Geometry: final body of the model. Coordinates: model frame, mm. Face numbers are marked on the shaded views. Round coordinates to 2 decimals unless told otherwise and drop trailing zeros. Write each loop counter-clockwise with the first axis right and the second up, starting at its lowest first coordinate (ties: lowest second). Pieces come first, ordered by that corner, then holes. Notation, with made-up numbers: (52.25, -34.5) - (58.25, -34.5) arc R20 cw to (58.25, -3.5) - close; hole circle Ø9 at (-27.5, 27.25). An arc over 180 degrees is marked (long way). Use a Markdown table: item, result. Add a question column.
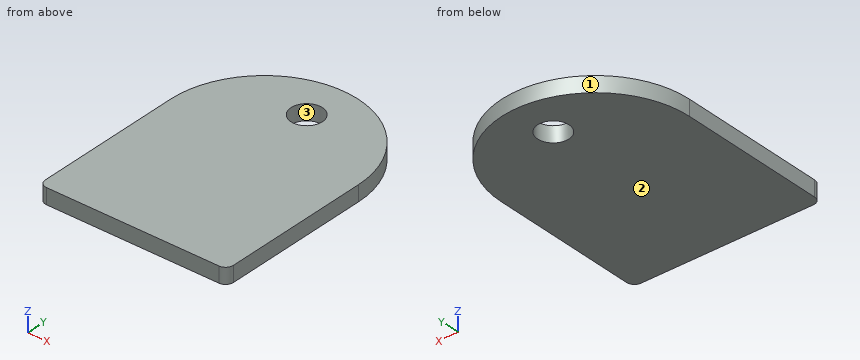
Autodesk Inventor part; units mm, degrees
ref_plane "YZ Plane" through (0, 0, 0) normal (1, 0, 0) x (0, 1, 0)
ref_plane "XZ Plane" through (0, 0, 0) normal (0, 1, 0) x (-1, 0, 0)
ref_plane "XY Plane" through (0, 0, 0) normal (0, 0, 1) x (1, 0, 0)
sketch "Sketch1" plane through (0, 0, 0) normal (0, 0, 1) x (1, 0, 0)
  circle A0 centre (-9.1291, -65.9913) radius 6.35
  line L0 (3.5709, -48.3129) -> (3.5709, -48.3129)
  line L1 (28.9709, -86.4129) -> (28.9709, -146.7379)
  line L2 (25.7959, -149.9129) -> (-44.0541, -149.9129)
  line L3 (-47.2291, -146.7379) -> (-47.2291, -86.4129)
  arc A1 (25.7959, -149.9129) -> (28.9709, -146.7379) centre (25.7959, -146.7379) ccw
  arc A2 (-47.2291, -146.7379) -> (-44.0541, -149.9129) centre (-44.0541, -146.7379) ccw
  line L4 (-9.1291, -48.3129) -> (-9.1291, -48.3129)
  arc A3 (-9.1291, -48.3129) -> (-47.2291, -86.4129) centre (-9.1291, -86.4129) ccw
  arc A4 (28.9709, -86.4129) -> (-9.1291, -48.3129) centre (-9.1291, -86.4129) ccw
  point P0 (0, 0)
  point P1 (28.9709, -149.9129)
  point P2 (-47.2291, -149.9129)
  point P3 (28.9709, -73.7129)
  dimension "d0" = 12.7
  dimension "d1" = 76.2
  dimension "d3" = 83.9216
  dimension "d4" = 38.1
  dimension "d11" = 101.6
  dimension "d12" = 38.1
extrude "Extrusion1" add sketch "Sketch1" along normal blind 6.35
properties part number "2 Stage Climer in a box lower bracket"
1) Section A-A, the plane x = -12.5. Return the cut outline in (y, z).
2) Draft query along X for the marked faces 1, 2 and 3. Return one class per face: released by +X, released by -X, zero draft, split by the parting line, or undercut.
3) Section C-C, the plane z = 4.25. Return the cut outline in (x, y) (3 decimals), then the cut area to 3 significant figures.
4) Pin query (flat end, axial travel): P1, Ø1.5, axis at x = -32, y = -85, coming from the -Z side; P2, Ø2, axis at y = -61, z = 2, coming from the -X side. Return the tip coordinate at first contact, or that it passes through.
5) Section D-D, the plane x = 4. Return the cut outline in (y, z), then the cut area to 3 significant figures.
6) Material intervals for L1, parallel to Y at x = -14, z = 4; L2, parallel to X at y = -60.5, z = 1; L3, parallel to X at y = -82.5, z = 4, sorted ascending. Write a range as from..to.
7) Section B-B, the plane y = -63.5. Return the cut outline in (x, z).
Output values:
| question | item | result |
|---|---|---|
| 1 | outline | (-149.91, 0) - (-71.37, 0) - (-71.37, 6.35) - (-149.91, 6.35) - close; (-60.61, 0) - (-48.46, 0) - (-48.46, 6.35) - (-60.61, 6.35) - close |
| 2 | face 1 | split by the parting line |
| 2 | face 2 | zero draft |
| 2 | face 3 | undercut |
| 3 | outline | (-47.229, -146.738) arc R3.175 ccw to (-44.054, -149.913) - (25.796, -149.913) arc R3.175 ccw to (28.971, -146.738) - (28.971, -86.413) arc R38.1 ccw to (-47.229, -86.413) - close; hole circle Ø12.7 at (-9.129, -65.991) |
| 3 | area | 6,990 mm^2 |
| 4 | P1 | stops at z = 0 |
| 4 | P2 | stops at x = -38.38 |
| 5 | outline | (-149.91, 0) - (-50.65, 0) - (-50.65, 6.35) - (-149.91, 6.35) - close |
| 5 | area | 630 mm^2 |
| 6 | L1 | y = -149.91..-70.07, -61.92..-48.63 |
| 6 | L2 | x = -37.06..-12.32, -5.94..18.8 |
| 6 | L3 | x = -47.03..28.77 |
| 7 | outline | (-39.57, 0) - (-14.97, 0) - (-14.97, 6.35) - (-39.57, 6.35) - close; (-3.29, 0) - (21.31, 0) - (21.31, 6.35) - (-3.29, 6.35) - close |
